Design review of the part built by this model. Coordinates are the model's own, in mm. A direction names the side the tool comes from. Round coordinates to 2 decimals unless told otherwise and drop trailing zeros. Loops run counter-clockwise (first coordinate to the right, second up) from the corner with the lowest first, then second, coordinate; pieces in that order, holes last. Notation, with made-up numbers: M 18,20 L 56,20 A20 ccw 56,57 Z; hole C -36.5,61 d11. An arc over 180 degrees is marked long. Answer as CSV lines item,"result". Start each with the question number.
Autodesk Inventor part; units mm, degrees
ref_plane "YZ Plane" through (0, 0, 0) normal (1, 0, 0) x (0, 1, 0)
ref_plane "XZ Plane" through (0, 0, 0) normal (0, 1, 0) x (-1, 0, 0)
ref_plane "XY Plane" through (0, 0, 0) normal (0, 0, 1) x (1, 0, 0)
sketch "Sketch1" plane through (0, 0, 0) normal (0, 0, 1) x (1, 0, 0)
  line L0 (0, 0) -> (83.6168, 0)
  line L1 (83.6168, 0) -> (83.6168, 85.7504)
  line L2 (83.6168, 85.7504) -> (0, 85.7504)
  line L3 (0, 85.7504) -> (0, 0)
  dimension "d0" = 83.6168
  dimension "d1" = 85.7504
extrude "Plate1" add sketch "Sketch1" along normal blind 3.048
sketch "Sketch2" plane through (83.6168, 3.048, 0) normal (0, -1, 0) x (1, 0, 0)
  line L0 (-83.6168, 0) -> (0, 0)
  line L1 (0, 0) -> (0, 25.4)
  line L2 (0, 25.4) -> (-83.6168, 25.4)
  line L3 (-83.6168, 25.4) -> (-83.6168, 0)
edge flange "Flange1" height 25.4 angle 90 thickness 3.048 bend radius 3.048 thickness toward (0, -1, 0) relief tear relief width 3.048 relief depth 1.524 edges at (41.8084, 0, 3.048) wall of the first edge with corners at (0, 3.048, 0) (83.6168, 3.048, 0) (83.6168, 3.048, 25.4) (0, 3.048, 25.4)
bend "Bend1"
corner "Corner1"
sketch "Sketch3" plane through (0, 0, 3.048) normal (0, 0, 1) x (1, 0, 0)
  line L0 (83.6168, 85.7504) -> (83.6168, 6.096)
  line L1 (0, 0) -> (83.6168, 0)
  point P0 (41.8084, 61.2902)
  dimension "d13" = 61.2902
  dimension "d14" = 41.8084
hole "Hole1" at (41.8084, 61.2902, 3.048) direction (0, 0, -1) diameter 26.1112 depth 3.048 tip angle 118
sketch "Sketch4" plane through (0, 0, 3.048) normal (0, 0, 1) x (1, 0, 0)
  circle A0 centre (41.8084, 61.2902) radius 13.0556
  point P0 (0, 0)
  point P1 (29.4386, 73.66)
  point P2 (54.1782, 73.66)
  point P3 (54.1782, 48.9204)
  point P4 (29.4386, 48.9204)
  dimension "d23" = 12.3698
  dimension "d24" = 12.3698
  dimension "d25" = 12.3698
  dimension "d26" = 12.3698
  dimension "d27" = 12.3698
  dimension "d28" = 12.3698
  dimension "d29" = 12.3698
  dimension "d30" = 12.3698
hole "Hole2" at (29.4386, 73.66, 3.048) at (54.1782, 73.66, 3.048) at (54.1782, 48.9204, 3.048) at (29.4386, 48.9204, 3.048) direction (0, 0, -1) diameter 4.2926 depth 3.048 tip angle 118
sketch "Sketch5" plane through (0, 3.048, 25.4) normal (0, 1, 0) x (1, 0, 0)
  line L0 (0, 0) -> (0, 19.304)
  point P0 (0, 25.4)
  point P1 (25.4, 9.652)
  point P2 (70.4595, 9.652)
  dimension "d39" = 25.4
hole "Hole3" at (25.4, 3.048, 15.748) at (70.4595, 3.048, 15.748) direction (0, -1, 0) diameter 6.35 end through all
equation "\"d20\" = Thickness"
equation "\"d36\" = Thickness"
equation "\"d45\" = Thickness"
equation "\"d3\" = BendReliefWidth"
equation "\"d4\" = BendReliefDepth"
equation "\"d5\" = MinimumRemnant"
equation "\"d6\" = BendRadius"
equation "\"d9\" = BendRadius"
equation "\"d10\" = CornerReliefSize"
equation "\"d11\" = GapSize"
equation "\"d12\" = JacobiRadiusSize"
equation "\"BendRadius\" = Thickness"
equation "\"BendReliefWidth\" = Thickness"
equation "\"BendReliefDepth\" = 0.5 * Thickness"
equation "\"CornerReliefSize\" = 4 * Thickness"
equation "\"MinimumRemnant\" = 2 * Thickness"
equation "\"TransitionRadius\" = BendRadius"
equation "\"JacobiRadiusSize\" = BendRadius"
equation "\"GapSize\" = Thickness"
equation "\"d2\" = BendRadius"
Item 1: To check wall thickness, follow line 1 (Z direction, x = 50.5, y = 48); line 2 (X direction, y = 64.5, z = 1.75). State the ranges of each line that lie inside material, in increasing order.
Item 2: The part is to be moulded in two halves that separate along Z. For faces 1 (the face through (42.39, 1.74, 1.83)), 2 (the face through (22.72, 1.5, 17.45)), 3 (the face through (41, 46, 3.048)), 4 (the face through (56.082, 47.93, 1.503)), say which applies: +Z half, -Z half, draft (parallel to the pull), parting line (faces both ways), or undercut.
Item 3: Consider section C-C, the plane z = 7.75. Write out the cut boundary in (x, y), then the cut area to 3 significant figures.
Item 4: Consider section A-A, the plane x = 25.4. Write out the cut boundary in (y, z), then the cut area to 3 significant figures.
Item 5: Insertion check: pin 1 Ø10 at (x, z) = (47, 19.5) entering from +Y; pin 2 Ø12 at (x, y) = (72.5, 76.5) entering from +Z; pin 3 Ø4 at (x, z) = (25.4, 15.748) entering from -Y; pin 4 Ø8 at (x, z) = (24.5, 10) entering from -Y. Each pin has a flat end and moves straight along its axis. Give the tip position at first contact, or say it passes through.
Item 6: Consider section B-B, the plane x = 64.5. Write out the cut boundary in (y, z), then the cut area to 3 significant figures.
Item 7: Tool access review of faces 5 (the face through (42, 3.048, 16)), 6 (the face through (28.794, 46.873, 1.503)): name each direction out of +Z, -Z, +X, -X, +Y, -Y from which nothing blocks a thin tool from reaching the whole face with its end or side.
Found:
1,line 1,"z = 0 to 3.05"
1,line 2,"x = 0 to 29.15, 54.46 to 83.62"
2,face 1,"-Z half"
2,face 2,"undercut"
2,face 3,"+Z half"
2,face 4,"draft"
3,outline,"M 0,0 L 83.62,0 L 83.62,3.05 L 0,3.05 Z"
3,area,"255 mm^2"
4,outline,"M 0,6.1 A6.1 ccw 6.1,0 L 85.75,0 L 85.75,3.05 L 6.1,3.05 A3.05 cw 3.05,6.1 L 3.05,12.57 L 0,12.57 Z; M 0,18.92 L 3.05,18.92 L 3.05,25.4 L 0,25.4 Z"
4,area,"304 mm^2"
5,pin 1,"stops at y = 3.05"
5,pin 2,"stops at z = 3.05"
5,pin 3,"passes through"
5,pin 4,"stops at y = 0"
6,outline,"M 0,6.1 A6.1 ccw 6.1,0 L 85.75,0 L 85.75,3.05 L 6.1,3.05 A3.05 cw 3.05,6.1 L 3.05,25.4 L 0,25.4 Z"
6,area,"324 mm^2"
7,face 5,"+Z, +X, -X, +Y"
7,face 6,"+Z, -Z"
